Could you check a few things on this drawing? It's one solid part, dimensions in mm from its lowest x, y, z. A direction names the side the tool comes from. Round coordinates to 2 decimals unless told otherwise and drop trailing zeros. Write each loop counter-clockwise with the first axis right and the second up, starting at its lowest first coordinate (ties: lowest second). Pieces come first, ordered by that corner, then holes. Notation, with made-up numbers: (39.5, 53.5) - (55.5, 53.5) arc R29 ccw to (55.5, 78.5) - close; hole circle Ø7 at (-30.5, -12.5). An arc over 180 degrees is marked (long way). Use one line per item in the form item = value. Start each with the question number.
1. If I drill on line 1 along Z through (x, y) = (6, 19.5); line 2 along X through (y, z) = (12.75, 84.5); line 3 along Y through (x, z) = (8.5, 31.5), over which ranges is the centre line in solid material (lowest first)?
2. Which directions (+Z, -Z, +X, -X, +Y, -Y) give clear straight access to the entire face, cutting with the end or side of a thin tool? Please do the marked faces 1 and 2.
3. Will these pins go through, and if not, where does the flat tip stop? pin 1 (1.5 mm diameter, centred on x = 21.5, y = 11, fed in from -Z); pin 2 (6 mm diameter, centred on x = 17.5, z = 65.5, fed in from +Y); pin 3 (5 mm diameter, centred on x = 7, z = 42.5, fed in from -Y); pin 4 (2 mm diameter, centred on x = 15, z = 37, fed in from -Y).
4. I want a section at D-D, the plane y = 7.25. List the corners of the cut face in (x, z) for me.
5. I want a section at A-A, the plane x = 12.5. List the corners of the cut face in (y, z) for me.
6. I want a section at C-C, the plane z = 98. List the corners of the cut face in (x, y) for me.
7. I want a section at B-B, the plane y = 12.5. List the corners of the cut face in (x, z) for me.
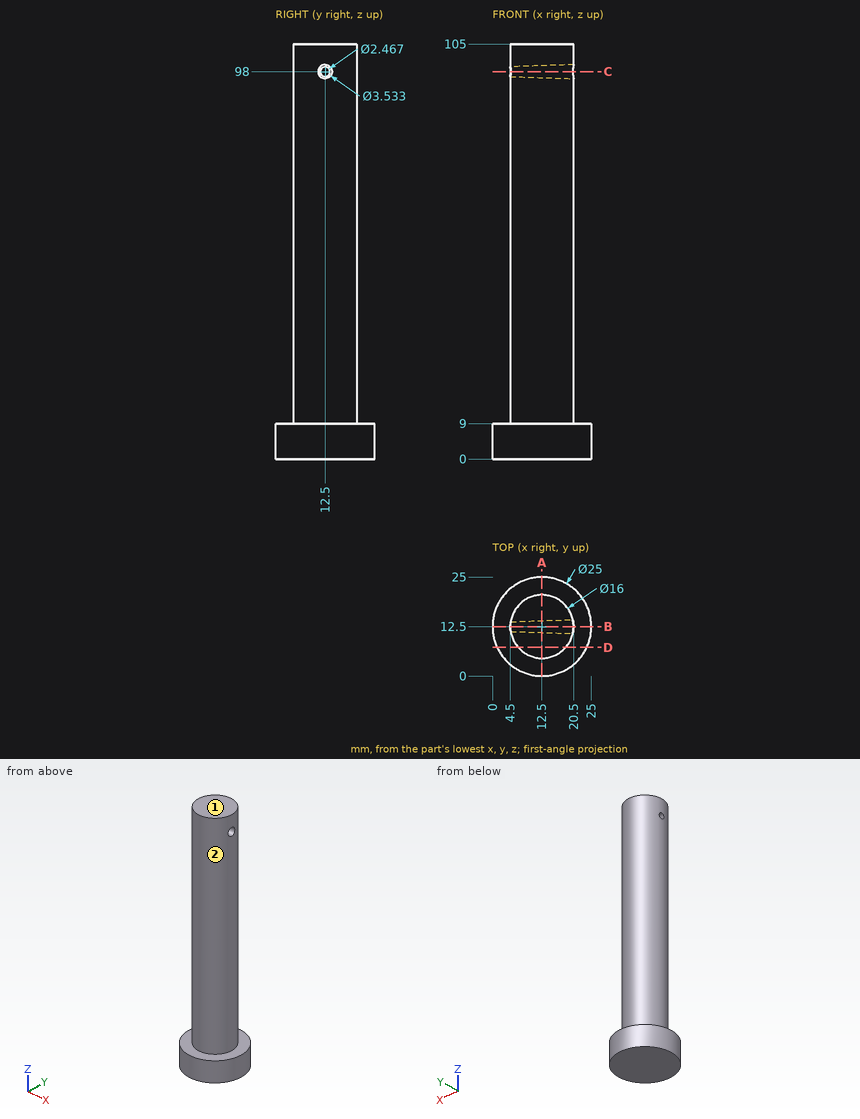
Model answer:
q1.line_1 = 0 to 9
q1.line_2 = 4.5 to 20.5
q1.line_3 = 5.57 to 19.43
q2.face_1 = +Z, +X, -X, +Y, -Y
q2.face_2 = +Z
q3.pin_1 = 0
q3.pin_2 = 20.25
q3.pin_3 = 5.08
q3.pin_4 = 4.64
q4.outline = (1.16, 0) - (23.84, 0) - (23.84, 9) - (18.54, 9) - (18.54, 105) - (6.46, 105) - (6.46, 9) - (1.16, 9) - close
q5.outline = (0, 0) - (25, 0) - (25, 9) - (20.5, 9) - (20.5, 105) - (4.5, 105) - (4.5, 9) - (0, 9) - close; hole circle Ø3 at (12.5, 98)
q6.outline = (4.6, 11.26) arc R8 ccw to (20.3, 10.74) - close; (4.6, 13.74) - (20.3, 14.26) arc R8 ccw to start
q7.outline = (0, 0) - (25, 0) - (25, 9) - (20.5, 9) - (20.5, 96.23) - (4.5, 96.77) - (4.5, 9) - (0, 9) - close; (4.5, 99.23) - (20.5, 99.77) - (20.5, 105) - (4.5, 105) - close
